```python
from build123d import *

# Parameters (mm, degrees)
ESQUISSE1_R                  = 115
BOSS_EXTRU_1_DEPTH           = 30
ESQUISSE4_R                  = 10
BOSS_EXTRU_3_DEPTH           = 60
ESQUISSE7_R                  = 8.5
BOSS_EXTRU_4_DEPTH           = 60
R_P_TITION_CIRCULAIRE1_COUNT = 3
ENL_V_START                  = -34
ESQUISSE8_R                  = 8.5
ESQUISSE8_R_2                = 7
ENL_V_MAT_EXTRU_1_DEPTH      = 1
ENL_V_START_2                = -5
ESQUISSE10_R                 = 105
ENL_V_MAT_EXTRU_2_DEPTH      = 20
ECHELLE1_SCALE               = 0.25


with BuildPart() as part:
    # Esquisse1 → Boss.-Extru.1 (new body)
    with BuildSketch(Plane.XY):
        Circle(ESQUISSE1_R)
        with BuildLine():
            Line((-90.226043394, -27.208254638), (-71.724215233, -16.583848882))
            ThreePointArc((-71.724215233, -16.583848882), (-33.409561028, 21.598796439), (-19.383519657, 73.840516299))
            Line((-19.383519657, 73.840516299), (-19.383519657, 93.840516299))
            ThreePointArc((-19.383519657, 93.840516299), (0, 113.224035956), (19.383519657, 93.840516299))
            Line((19.383519657, 93.840516299), (19.383519657, 73.840516299))
            ThreePointArc((19.383519657, 73.840516299), (33.739018197, 20.139465346), (72.975743183, -19.235179086))
            Line((72.975743183, -19.235179086), (90.272811294, -29.275668854))
            ThreePointArc((90.272811294, -29.275668854), (97.529389636, -56.613226732), (70.191831757, -63.869805074))
            Line((70.191831757, -63.869805074), (52.894763647, -53.829315306))
            ThreePointArc((52.894763647, -53.829315306), (1.242076374, -39.859433821), (-50.47540372, -53.587505203))
            Line((-50.47540372, -53.587505203), (-68.97723188, -64.211910959))
            ThreePointArc((-68.97723188, -64.211910959), (-98.103465797, -56.334488555), (-90.226043394, -27.208254638))
        make_face(mode=Mode.SUBTRACT)
    extrude(amount=BOSS_EXTRU_1_DEPTH)

    # Esquisse4 → Boss.-Extru.3 (add)
    with BuildSketch(Plane.XY):
        with BuildLine():
            Line((-90.226043394, -27.208254638), (-71.724215233, -16.583848882))
            ThreePointArc((-71.724215233, -16.583848882), (-33.409561028, 21.598796439), (-19.383519657, 73.840516299))
            Line((-19.383519657, 73.840516299), (-19.383519657, 93.840516299))
            ThreePointArc((-19.383519657, 93.840516299), (0, 113.224035956), (19.383519657, 93.840516299))
            Line((19.383519657, 93.840516299), (19.383519657, 73.840516299))
            ThreePointArc((19.383519657, 73.840516299), (33.739018197, 20.139465346), (72.975743183, -19.235179086))
            Line((72.975743183, -19.235179086), (90.272811294, -29.275668854))
            ThreePointArc((90.272811294, -29.275668854), (97.529389636, -56.613226732), (70.191831757, -63.869805074))
            Line((70.191831757, -63.869805074), (52.894763647, -53.829315306))
            ThreePointArc((52.894763647, -53.829315306), (1.242076374, -39.859433821), (-50.47540372, -53.587505203))
            Line((-50.47540372, -53.587505203), (-68.97723188, -64.211910959))
            ThreePointArc((-68.97723188, -64.211910959), (-98.103465797, -56.334488555), (-90.226043394, -27.208254638))
        make_face()
        with Locations(Location((0, 0, 0), (0, 0, 180))):
            Circle(ESQUISSE4_R, mode=Mode.SUBTRACT)
    extrude(amount=BOSS_EXTRU_3_DEPTH)

    # Esquisse7 → Boss.-Extru.4 (add)
    with BuildSketch(Plane.XY.offset(60)):
        with Locations(Location((0, 72, 0), (0, 0, 180))):
            Circle(ESQUISSE7_R)
    boss_extru_4 = extrude(amount=BOSS_EXTRU_4_DEPTH)

    # Répétition circulaire1: Boss.-Extru.4 ×3 about axis
    r_p_tition_circulaire1_axis = Axis((0, 0, 0), (0, 0, 1))
    for i in range(1, R_P_TITION_CIRCULAIRE1_COUNT):
        add(boss_extru_4.rotate(r_p_tition_circulaire1_axis, i * 360 / R_P_TITION_CIRCULAIRE1_COUNT))

    # Esquisse8 → Enlèv. mat.-Extru.1 (cut)
    # profile 1 of 3: a face of its own
    with BuildSketch(Plane.XY.offset(120).offset(ENL_V_START)):
        with Locations(Location((0, 72, 0), (0, 0, 180))):
            Circle(ESQUISSE8_R)
        with Locations((0, 72)):
            Circle(ESQUISSE8_R_2, mode=Mode.SUBTRACT)
    # profile 2 of 3: a face of its own
    with BuildSketch(Plane.XY.offset(120).offset(ENL_V_START)):
        with Locations((-62.437871739, -35.854039838)):
            Circle(ESQUISSE8_R)
        with Locations((-62.437871739, -35.854039838)):
            Circle(ESQUISSE8_R_2, mode=Mode.SUBTRACT)
    # profile 3 of 3: a face of its own
    with BuildSketch(Plane.XY.offset(120).offset(ENL_V_START)):
        with Locations(Location((62.353829072, -36, 0), (0, 0, 180))):
            Circle(ESQUISSE8_R)
        with Locations((62.353829072, -36)):
            Circle(ESQUISSE8_R_2, mode=Mode.SUBTRACT)
    extrude(amount=ENL_V_MAT_EXTRU_1_DEPTH, mode=Mode.SUBTRACT)

    # Esquisse10 → Enlèv. mat.-Extru.2 (cut)
    with BuildSketch(Plane(origin=(0, 0, 0), x_dir=(-1, 0, 0), z_dir=(0, 0, -1)).offset(ENL_V_START_2)):
        Circle(ESQUISSE10_R)
    extrude(amount=-ENL_V_MAT_EXTRU_2_DEPTH, mode=Mode.SUBTRACT)


with BuildPart() as part_1:
    # Echelle1: scaled about (-0.37502274, -0.313761963, 30.457504843)
    add(part.part.scale(ECHELLE1_SCALE).moved(Location((-0.281267055, -0.235321472, 22.843128632))))


solid = part_1.part
```
The listing builds one solid part. Answer for the finished solid, in the listing's coordinates (mm). A direction names the side the tool comes from. Coordinates: 2 decimals unless noted, no trailing zeros. Write each loop counter-clockwise with the first axis right and the second up, starting at its lowest first coordinate (ties: lowest second). Pieces come first, ordered by that corner, then holes. Notation, with made-up numbers: M -33,56 L -8,56 A7 ccw -8,68 Z; hole C 24,62.5 d8. An arc over 180 degrees is marked long. Use a Markdown table: item, result. Add a question column.
1. Given P1, Ø4, axis at y = 21.5, z = 33, coming from the +X side; P2, Ø8, axis at x = -0.28, y = -0.24, coming from the -Z side; P3, Ø22.5, axis at x = 0.5, y = -4, coming from the +Z side; P4, Ø2, axis at x = -9.5, z = 38.5, coming from the +Y side, each flat-ended and moving along its own axis, determine where each tip first touches the part or whether it passes through.
2. For a pull along X with two mould halves and no side action, classify faces 1 (the cylindrical face through (8.056, 4.97, 34.041)), 2 (the cylindrical face through (0.2, -10.2, 34)), 3 (the flat face through (0, 18, 52.843)) as +X half, -X half, draft (parallel to the pull), parting line (faces both ways), or undercut.
3. Section B-B (y = 11) is taken. Give the vertices of the cut face in (x, z).
4. Which of the six approach directions +Z, -Z, +X, -X, +Y, -Y give full straight-line access (tool end or side, diameter ignored) to faces 4 (the flat face through (-15.18, -14.94, 34.04)), 5 (the cylindrical face through (-0.39, 28.07, 34.04)), 6 (the flat face through (-14, -9, 44.593)), 7 (the cylindrical face through (-2.3, 17.1, 41))?
5. Section A-A (x = 24) is taken. Give the vertices of the cut face in (y, z), plus the area to 3 significant figures.
6. Section C-C (z = 43.5) is taken. Give the vertices of the cut face in (x, y) (3 decimals).
7. Straight lines are drawn through the part: line 1 along Z through (x, y) = (12.5, -3.5); line 2 along Z through (x, y) = (20.5, 12); line 3 along X through (y, z) = (-17.5, 26). For each, find the intervals that lie inside material, in ascending order. Write a range as [from, to].
8. Section D-D (y = -24.5) is taken. Give the vertices of the cut face in (x, z).
Data:
| question | item | result |
|---|---|---|
| 1 | P1 | stops at x = 4.56 |
| 1 | P2 | stops at z = 22.84 |
| 1 | P3 | stops at z = 37.84 |
| 1 | P4 | stops at y = 4.97 |
| 2 | face 1 | +X half |
| 2 | face 2 | undercut |
| 2 | face 3 | draft |
| 3 | outline | M -26.75,22.84 L 26.18,22.84 L 26.18,30.34 L 5.55,30.34 L 5.55,37.84 L -6.15,37.84 L -6.15,30.34 L -26.75,30.34 Z; hole M -24.01,24.09 L 23.44,24.09 L 23.44,29.09 L -24.01,29.09 Z |
| 4 | face 4 | +Z, -Y |
| 4 | face 5 | +Z, +Y |
| 4 | face 6 | none |
| 4 | face 7 | +Z |
| 5 | outline | M -15.63,22.84 L 15.16,22.84 L 15.16,30.34 L -9.2,30.34 L -9.2,37.84 L -14.56,37.84 L -14.56,30.34 L -15.63,30.34 Z; hole M -10.21,24.09 L 9.74,24.09 L 9.74,29.09 L -10.21,29.09 Z |
| 5 | area | 171 mm2 |
| 6 | outline | C -15.87,-9.235 d4.25; C -0.281,17.765 d4.25; C 15.307,-9.235 d4.25 |
| 7 | line 1 | z = [22.84, 24.09], [29.09, 37.84] |
| 7 | line 2 | z = [22.84, 24.09], [29.09, 30.34] |
| 7 | line 3 | x = [-23.27, -20.05], [19.49, 22.71] |
| 8 | outline | M -15.7,22.84 L 15.14,22.84 L 15.14,30.34 L -15.7,30.34 Z; hole M -10.3,24.09 L 9.73,24.09 L 9.73,29.09 L -10.3,29.09 Z |
